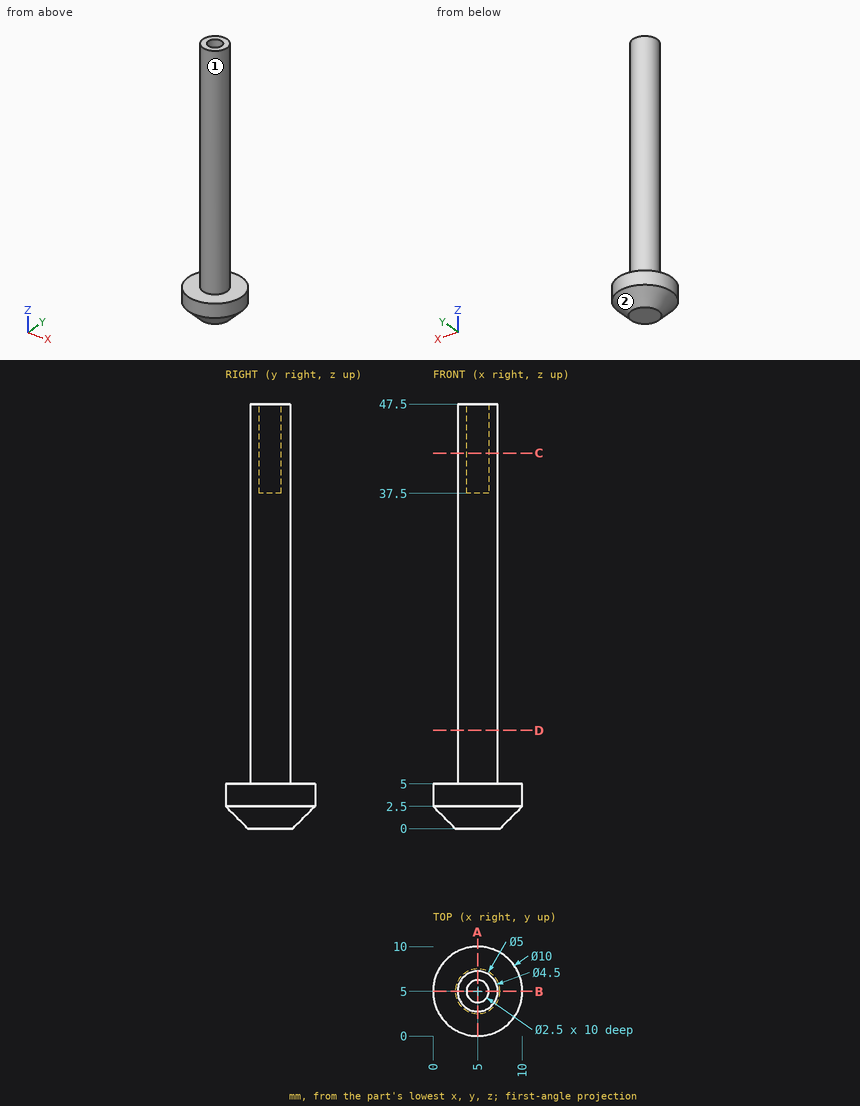
Design review of the part shown in the three views and the two pictorial views. Dimensions are in mm from the part's minimum x, y and z. A direction names the side the tool comes from. Round coordinates to 2 decimals unless told otherwise and drop trailing zeros. Write each loop counter-clockwise with the first axis right and the second up, starting at its lowest first coordinate (ties: lowest second). Pieces come first, ordered by that corner, then holes.
1) For line 1 along Y through (x, z) = (5, 41.75); line 2 along Z through (x, y) = (5.25, 4); line 3 along Z through (x, y) = (8.5, 6.5), list the stretches that pass through material, from the lowest coordinate up.
Answer below:
line 1: y = 2.75 to 3.75, 6.25 to 7.25
line 2: z = 0 to 37.5
line 3: z = 1.31 to 5
2) Take a section at D-D on z = 11. Give the boundary of the cut face in (x, y), then the cut area to 3 significant figures.
Answer below:
outline: circle Ø4.5 at (5, 5)
area: 15.9 mm2
3) Insertion check: pin 1 Ø1.5 at (x, y) = (5, 5) entering from +Z; pin 2 Ø1 at (x, z) = (3, 42.5) entering from +Y; pin 3 Ø3 at (y, z) = (3, 30.5) entering from +X; pin 4 Ø4 at (x, y) = (5.5, 6) entering from +Z. Each pin has a flat end and moves straight along its axis. Give the tip position at first contact, or say it passes through.
Answer below:
pin 1: stops at z = 37.5
pin 2: stops at y = 6.68
pin 3: stops at x = 7.19
pin 4: stops at z = 47.5
4) Machinability: for the marked faces 1 and 2, which of the approach directions +Z, -Z, +X, -X, +Y, -Y give a long, thin tool a straight path to every point of the face, cutting with its end or side? Answer none if there is none.
Answer below:
face 1: +Z
face 2: -Z
5) Take a section at A-A on x = 5. Give the boundary of the cut face in (y, z).
Answer below:
outline: (0, 2.5) - (2.5, 0) - (7.5, 0) - (10, 2.5) - (10, 5) - (7.25, 5) - (7.25, 47.5) - (6.25, 47.5) - (6.25, 37.5) - (3.75, 37.5) - (3.75, 47.5) - (2.75, 47.5) - (2.75, 5) - (0, 5) - close
6) Take a section at C-C on z = 42. Give the boundary of the cut face in (x, y), then the cut area to 3 significant figures.
Answer below:
outline: circle Ø4.5 at (5, 5); hole circle Ø2.5 at (5, 5)
area: 11.0 mm2
